Can you work these out from the model? Positions are in its coordinate system, mm. Give positions to 0.01 mm unless a question says otherwise; leave off trailing zeros. Write each loop counter-clockwise with the first axis right and the second up, starting at its lowest first coordinate (ties: lowest second). Pieces come first, ordered by that corner, then holes. Notation, with made-up numbers: (53.25, -39) -> (58.25, -39) arc R20 cw to (58.25, -9) -> close; hole circle Ø7 at (-10, 48.25). An arc over 180 degrees is marked (long way). One line per item, written item: value.
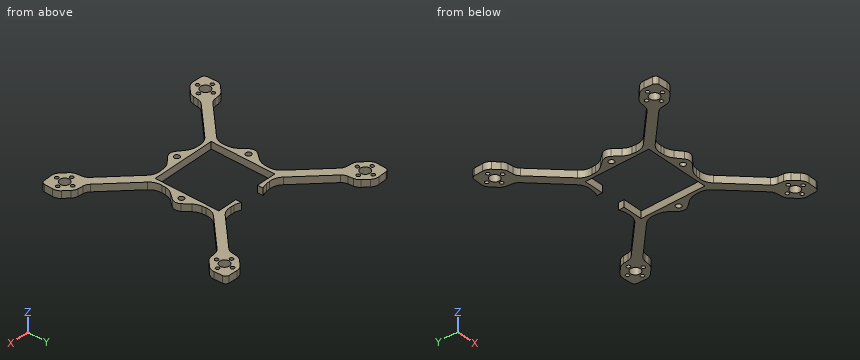
from build123d import *

# Parameters (mm, degrees)
F0_R     = 1
F0_R_2   = 2.75
F0_R_3   = 1.5
F1_DEPTH = 4


with BuildPart() as f1:
    # F0 (on Top) → F1 (new body)
    with BuildSketch(Plane.XY):
        with BuildLine():
            Line((-18, -18), (-18, 18))
            Line((-18, 18), (-7, 18))
            Line((-7, 18), (-7, 21.136517))
            ThreePointArc((-7, 21.136517), (-8.652636, 20.40417), (-10.427502, 20.061548))
            Line((-10.427502, 20.061548), (-12.414831, 19.907267))
            ThreePointArc((-12.414831, 19.907267), (-15.806951, 20.37921), (-18.69088, 22.226414))
            Line((-18.69088, 22.226414), (-35.882908, 39.418442))
            ThreePointArc((-35.882908, 39.418442), (-36.85389, 40.788032), (-37.316792, 42.401818))
            Line((-37.316792, 42.401818), (-37.636526, 45.279423))
            ThreePointArc((-37.636526, 45.279423), (-38.099429, 46.893209), (-39.070411, 48.262799))
            Line((-39.070411, 48.262799), (-41.9391, 51.131488))
            ThreePointArc((-41.9391, 51.131488), (-43.653931, 52.252674), (-45.674474, 52.591959))
            Line((-45.674474, 52.591959), (-50.481223, 52.399689))
            ThreePointArc((-50.481223, 52.399689), (-51.815501, 51.815501), (-52.399689, 50.481223))
            Line((-52.399689, 50.481223), (-52.591959, 45.674474))
            ThreePointArc((-52.591959, 45.674474), (-52.252674, 43.653931), (-51.131488, 41.9391))
            Line((-51.131488, 41.9391), (-48.262799, 39.070411))
            ThreePointArc((-48.262799, 39.070411), (-46.893209, 38.099429), (-45.279423, 37.636526))
            Line((-45.279423, 37.636526), (-42.401818, 37.316792))
            ThreePointArc((-42.401818, 37.316792), (-40.788032, 36.85389), (-39.418442, 35.882908))
            Line((-39.418442, 35.882908), (-22.226414, 18.69088))
            ThreePointArc((-22.226414, 18.69088), (-20.37921, 15.806951), (-19.907267, 12.414831))
            Line((-19.907267, 12.414831), (-20.061548, 10.427502))
            ThreePointArc((-20.061548, 10.427502), (-20.58741, 8.132004), (-21.758856, 6.089075))
            Line((-21.758856, 6.089075), (-24.646599, 2.431827))
            ThreePointArc((-24.646599, 2.431827), (-25.49094, 0), (-24.646599, -2.431827))
            Line((-24.646599, -2.431827), (-21.758856, -6.089075))
            ThreePointArc((-21.758856, -6.089075), (-20.58741, -8.132004), (-20.061548, -10.427502))
            Line((-20.061548, -10.427502), (-19.907267, -12.414831))
            ThreePointArc((-19.907267, -12.414831), (-20.37921, -15.806951), (-22.226414, -18.69088))
            Line((-22.226414, -18.69088), (-39.418442, -35.882908))
            ThreePointArc((-39.418442, -35.882908), (-40.788032, -36.85389), (-42.401818, -37.316792))
            Line((-42.401818, -37.316792), (-45.279423, -37.636526))
            ThreePointArc((-45.279423, -37.636526), (-46.893209, -38.099429), (-48.262799, -39.070411))
            Line((-48.262799, -39.070411), (-51.131488, -41.9391))
            ThreePointArc((-51.131488, -41.9391), (-52.252674, -43.653931), (-52.591959, -45.674474))
            Line((-52.591959, -45.674474), (-52.399689, -50.481223))
            ThreePointArc((-52.399689, -50.481223), (-51.815501, -51.815501), (-50.481223, -52.399689))
            Line((-50.481223, -52.399689), (-45.674474, -52.591959))
            ThreePointArc((-45.674474, -52.591959), (-43.653931, -52.252674), (-41.9391, -51.131488))
            Line((-41.9391, -51.131488), (-39.070411, -48.262799))
            ThreePointArc((-39.070411, -48.262799), (-38.099429, -46.893209), (-37.636526, -45.279423))
            Line((-37.636526, -45.279423), (-37.316792, -42.401818))
            ThreePointArc((-37.316792, -42.401818), (-36.85389, -40.788032), (-35.882908, -39.418442))
            Line((-35.882908, -39.418442), (-18.69088, -22.226414))
            ThreePointArc((-18.69088, -22.226414), (-15.806951, -20.37921), (-12.414831, -19.907267))
            Line((-12.414831, -19.907267), (-10.427502, -20.061548))
            ThreePointArc((-10.427502, -20.061548), (-8.132004, -20.58741), (-6.089075, -21.758856))
            Line((-6.089075, -21.758856), (-2.431827, -24.646599))
            ThreePointArc((-2.431827, -24.646599), (0, -25.49094), (2.431827, -24.646599))
            Line((2.431827, -24.646599), (6.089075, -21.758856))
            ThreePointArc((6.089075, -21.758856), (8.132004, -20.58741), (10.427502, -20.061548))
            Line((10.427502, -20.061548), (12.414831, -19.907267))
            ThreePointArc((12.414831, -19.907267), (15.806951, -20.37921), (18.69088, -22.226414))
            Line((18.69088, -22.226414), (35.882908, -39.418442))
            ThreePointArc((35.882908, -39.418442), (36.85389, -40.788032), (37.316792, -42.401818))
            Line((37.316792, -42.401818), (37.636526, -45.279423))
            ThreePointArc((37.636526, -45.279423), (38.099429, -46.893209), (39.070411, -48.262799))
            Line((39.070411, -48.262799), (41.9391, -51.131488))
            ThreePointArc((41.9391, -51.131488), (43.653931, -52.252674), (45.674474, -52.591959))
            Line((45.674474, -52.591959), (50.481223, -52.399689))
            ThreePointArc((50.481223, -52.399689), (51.815501, -51.815501), (52.399689, -50.481223))
            Line((52.399689, -50.481223), (52.591959, -45.674474))
            ThreePointArc((52.591959, -45.674474), (52.252674, -43.653931), (51.131488, -41.9391))
            Line((51.131488, -41.9391), (48.262799, -39.070411))
            ThreePointArc((48.262799, -39.070411), (46.893209, -38.099429), (45.279423, -37.636526))
            Line((45.279423, -37.636526), (42.401818, -37.316792))
            ThreePointArc((42.401818, -37.316792), (40.788032, -36.85389), (39.418442, -35.882908))
            Line((39.418442, -35.882908), (22.226414, -18.69088))
            ThreePointArc((22.226414, -18.69088), (20.37921, -15.806951), (19.907267, -12.414831))
            Line((19.907267, -12.414831), (20.061548, -10.427502))
            ThreePointArc((20.061548, -10.427502), (20.58741, -8.132004), (21.758856, -6.089075))
            Line((21.758856, -6.089075), (24.646599, -2.431827))
            ThreePointArc((24.646599, -2.431827), (25.49094, 0), (24.646599, 2.431827))
            Line((24.646599, 2.431827), (21.758856, 6.089075))
            ThreePointArc((21.758856, 6.089075), (20.58741, 8.132004), (20.061548, 10.427502))
            Line((20.061548, 10.427502), (19.907267, 12.414831))
            ThreePointArc((19.907267, 12.414831), (20.37921, 15.806951), (22.226414, 18.69088))
            Line((22.226414, 18.69088), (39.418442, 35.882908))
            ThreePointArc((39.418442, 35.882908), (40.788032, 36.85389), (42.401818, 37.316792))
            Line((42.401818, 37.316792), (45.279423, 37.636526))
            ThreePointArc((45.279423, 37.636526), (46.893209, 38.099429), (48.262799, 39.070411))
            Line((48.262799, 39.070411), (51.131488, 41.9391))
            ThreePointArc((51.131488, 41.9391), (52.252674, 43.653931), (52.591959, 45.674474))
            Line((52.591959, 45.674474), (52.399689, 50.481223))
            ThreePointArc((52.399689, 50.481223), (51.815501, 51.815501), (50.481223, 52.399689))
            Line((50.481223, 52.399689), (45.674474, 52.591959))
            ThreePointArc((45.674474, 52.591959), (43.653931, 52.252674), (41.9391, 51.131488))
            Line((41.9391, 51.131488), (39.070411, 48.262799))
            ThreePointArc((39.070411, 48.262799), (38.099429, 46.893209), (37.636526, 45.279423))
            Line((37.636526, 45.279423), (37.316792, 42.401818))
            ThreePointArc((37.316792, 42.401818), (36.85389, 40.788032), (35.882908, 39.418442))
            Line((35.882908, 39.418442), (18.69088, 22.226414))
            ThreePointArc((18.69088, 22.226414), (15.806951, 20.37921), (12.414831, 19.907267))
            Line((12.414831, 19.907267), (10.427502, 20.061548))
            ThreePointArc((10.427502, 20.061548), (8.652636, 20.40417), (7, 21.136517))
            Line((7, 21.136517), (7, 18))
            Line((7, 18), (18, 18))
            Line((18, 18), (18, -18))
            Line((18, -18), (-18, -18))
        make_face()
        with Locations((-45.254834, -49.754834)):
            Circle(F0_R, mode=Mode.SUBTRACT)
        with Locations((-49.754834, -45.254834)):
            Circle(F0_R, mode=Mode.SUBTRACT)
        with Locations((-45.254834, -45.254834)):
            Circle(F0_R_2, mode=Mode.SUBTRACT)
        with Locations((-40.754834, -45.254834)):
            Circle(F0_R, mode=Mode.SUBTRACT)
        with Locations((-45.254834, -40.754834)):
            Circle(F0_R, mode=Mode.SUBTRACT)
        with Locations((45.254834, -49.754834)):
            Circle(F0_R, mode=Mode.SUBTRACT)
        with Locations((40.754834, -45.254834)):
            Circle(F0_R, mode=Mode.SUBTRACT)
        with Locations((45.254834, -45.254834)):
            Circle(F0_R_2, mode=Mode.SUBTRACT)
        with Locations((45.254834, -40.754834)):
            Circle(F0_R, mode=Mode.SUBTRACT)
        with Locations((49.754834, -45.254834)):
            Circle(F0_R, mode=Mode.SUBTRACT)
        with Locations((0, -21.566757)):
            Circle(F0_R_3, mode=Mode.SUBTRACT)
        with Locations((-21.566757, 0)):
            Circle(F0_R_3, mode=Mode.SUBTRACT)
        with Locations((-49.754834, 45.254834)):
            Circle(F0_R, mode=Mode.SUBTRACT)
        with Locations((-45.254834, 40.754834)):
            Circle(F0_R, mode=Mode.SUBTRACT)
        with Locations((-45.254834, 45.254834)):
            Circle(F0_R_2, mode=Mode.SUBTRACT)
        with Locations((-40.754834, 45.254834)):
            Circle(F0_R, mode=Mode.SUBTRACT)
        with Locations((-45.254834, 49.754834)):
            Circle(F0_R, mode=Mode.SUBTRACT)
        with Locations((21.566757, 0)):
            Circle(F0_R_3, mode=Mode.SUBTRACT)
        with Locations((45.254834, 40.754834)):
            Circle(F0_R, mode=Mode.SUBTRACT)
        with Locations((40.754834, 45.254834)):
            Circle(F0_R, mode=Mode.SUBTRACT)
        with Locations((45.254834, 45.254834)):
            Circle(F0_R_2, mode=Mode.SUBTRACT)
        with Locations((49.754834, 45.254834)):
            Circle(F0_R, mode=Mode.SUBTRACT)
        with Locations((45.254834, 49.754834)):
            Circle(F0_R, mode=Mode.SUBTRACT)
    extrude(amount=F1_DEPTH)


solid = f1.part
1) Will these pins go through, and if not, where does the flat tip stop? pin 1 (2.5 mm diameter, centred on x = 21.57, y = 0, fed in from -Z); pin 2 (1.2 mm diameter, centred on y = 2, z = 2, fed in from +X); pin 3 (2 mm diameter, centred on x = -12.5, z = 2.5, fed in from -Y); pin 4 (1.5 mm diameter, centred on x = -35.5, z = 3.5, fed in from +Y).
Answer list:
pin 1: passes through
pin 2: stops at x = 25.23
pin 3: stops at y = -19.98
pin 4: stops at y = 39.83
2) If we section it at A-A (y = 0): Write out the boundary of the cut face in (x, z).
Answer list:
outline: (-25.49, 0) -> (-23.07, 0) -> (-23.07, 4) -> (-25.49, 4) -> close; (-20.07, 0) -> (-18, 0) -> (-18, 4) -> (-20.07, 4) -> close; (18, 0) -> (20.07, 0) -> (20.07, 4) -> (18, 4) -> close; (23.07, 0) -> (25.49, 0) -> (25.49, 4) -> (23.07, 4) -> close
3) If we section it at B-B (x = 0): Write out the boundary of the cut face in (y, z), and give its area (3 significant figures).
Answer list:
outline: (-25.49, 0) -> (-23.07, 0) -> (-23.07, 4) -> (-25.49, 4) -> close; (-20.07, 0) -> (-18, 0) -> (-18, 4) -> (-20.07, 4) -> close
area: 18.0 mm^2
4) If we section it at D-D (z = 3): State how many separate pieces and enclosed holes the cut face has, and give its area (3 significant figures).
Answer list:
separate pieces: 1
enclosed holes: 23
area: 1,590 mm^2
5) If we section it at C-C (y = 28): Write out the boundary of the cut face in (x, z), and give its area (3 significant figures).
Answer list:
outline: (-31.54, 0) -> (-24.46, 0) -> (-24.46, 4) -> (-31.54, 4) -> close; (24.46, 0) -> (31.54, 0) -> (31.54, 4) -> (24.46, 4) -> close
area: 56.6 mm^2
6) I need wall thicknesses on L1, parallel to X at y = -40.5, z = 1.5; L2, parallel to Y at x = -21, z = 1.3; L3, parallel to Y at x = 25, z = 3.3. Which ranges of each line are inside material? Lowest first, please.
Answer list:
L1: x = -49.69 to -46.22, -44.29 to -36.7, 36.7 to 44.29, 46.22 to 49.69
L2: y = -24.54 to -17.11, -7.24 to -1.39, 1.39 to 7.24, 17.11 to 24.54
L3: y = -28.54 to -21.46, -1.9 to 1.9, 21.46 to 28.54
